Autodesk Fusion 360 part; units mm, degrees
sketch "Sketch1" plane through (0, 0, 0) normal (0, 1, 0) x (1, 0, 0)
  circle A0 centre (0, 96.75) radius 3
  arc A1 (12.5, 96.75) -> (-12.5, 96.75) centre (0, 96.75) ccw
  line L0 (12.5, 96.75) -> (12.5, -53.25)
  arc A2 (-12.5, -53.25) -> (12.5, -53.25) centre (0, -53.25) ccw
  line L1 (-12.5, -53.25) -> (-12.5, 96.75)
  circle A3 centre (0, -53.25) radius 3
  point P0 (-35.6168, 0)
extrude "Extrude1" add sketch "Sketch1" along normal blind 6
The model under review builds one solid part; all positions refer to its coordinate system, in mm. Round coordinates to 2 decimals unless told otherwise and drop trailing zeros. Write each loop counter-clockwise with the first axis right and the second up, starting at its lowest first coordinate (ties: lowest second). Pieces come first, ordered by that corner, then holes. Notation, with made-up numbers: M 78.25,36.25 L 133.25,36.25 A19 cw 133.25,73.25 Z; hole C 46,85 d9. An arc over 180 degrees is marked long. Use a Markdown table: item, result. Add a question column.
Q1. Insertion check: pin 1 (1 mm diameter, centred on x = 5.5, y = 2, fed in from -Z). The pin has a flat end and moves straight along its axis. Give the tip position at first contact, or say it passes through.
Q2. We need section B-B, the plane y = 4.6. State the section outline as (x, z) points, plus the area to 3 significant figures.
Q3. The part is to be moulded in two halves that separate along Z. For faces 1 (the face through (0, 0, -23)), 2 (the face through (-0.391, 2.958, 56.224)), 3 (the face through (-0.275, 2.958, -109.247)), say which applies: pulls with the +Z half, pulls with the -Z half, needs draft (parallel to the pull), parting line crosses it, or undercut.
Q4. To check wall thickness, follow line 1 (Z direction, x = 0, y = 1.65); line 2 (X direction, y = 3.15, z = -96.75); line 3 (Z direction, x = -1.75, y = 3.95). State the ranges of each line that lie inside material, in increasing order.
Q5. We need section C-C, the plane x = -7. State the section outline as (y, z) points, plus the area to 3 significant figures.
Q6. We need section A-A, the plane x = 0. State the section outline as (y, z) points.
Findings below:
| question | item | result |
|---|---|---|
| 1 | pin 1 | stops at z = -108.21 |
| 2 | outline | M -12.5,-96.75 A12.5 ccw 12.5,-96.75 L 12.5,53.25 A12.5 ccw -12.5,53.25 Z; hole C 0,-96.75 d6; hole C 0,53.25 d6 |
| 2 | area | 4,180 mm² |
| 3 | face 1 | needs draft |
| 3 | face 2 | undercut |
| 3 | face 3 | pulls with the -Z half |
| 4 | line 1 | z = -109.25 to -99.75, -93.75 to 50.25, 56.25 to 65.75 |
| 4 | line 2 | x = -12.5 to -3, 3 to 12.5 |
| 4 | line 3 | z = -109.13 to -99.19, -94.31 to 50.81, 55.69 to 65.63 |
| 5 | outline | M 0,-107.11 L 6,-107.11 L 6,63.61 L 0,63.61 Z |
| 5 | area | 1,020 mm² |
| 6 | outline | M 0,-109.25 L 6,-109.25 L 6,-99.75 L 0,-99.75 Z; M 0,-93.75 L 6,-93.75 L 6,50.25 L 0,50.25 Z; M 0,56.25 L 6,56.25 L 6,65.75 L 0,65.75 Z |
